Source: CAD feature listing. Evaluate the final solid. Frame: model axes, mm. A direction names the side the tool comes from. Give positions to 0.01 mm unless a question says otherwise; leave off trailing zeros. Write each loop counter-clockwise with the first axis right and the second up, starting at its lowest first coordinate (ties: lowest second). Pieces come first, ordered by that corner, then holes. Notation, with made-up numbers: (-19.75, 19.5) -> (27.25, 19.5) arc R19 cw to (27.25, 41.5) -> close; hole circle Ø2 at (16.25, 62). An arc over 180 degrees is marked (long way). Answer as a JSON object with one key per item and string values. Group by question number.
Item 1: First-contact query: pin 1 Ø4 at (x, z) = (10.26, -4.32) entering from +Y; pin 2 Ø17.5 at (x, z) = (-20, 9) entering from -Y; pin 3 Ø2 at (x, y) = (-0.5, 2.5) entering from +Z; pin 4 Ø6 at (y, z) = (-10, 9.5) entering from -X. Flat tips, straight axial feed; report the tip coordinate or a pass-through.
Item 2: Section query A-A on z = 0. Return the cut outline in (x, y).
Item 3: Access query for faces 5 (the face through (-16, 0, 12)), 6 (the face through (-11, 4, 18.368)), 7 (the face through (-15, 4, -9.832)), 8 (the face through (-16, 7.2, 12)). Directions: +Z, -Z, +X, -X, +Y, -Y. A direction counts if a zero-diameter tool reaches every point of the face in a straight line with its end or side. Return the directions, or none.
Item 4: Section query B-B on x = 2. Return the cut outline in (y, z), plus the area to 3 significant figures.
Item 5: Pull-direction query (X, two-part tool) for faces 1 (the face through (-35.136, 4, 1)), 2 (the face through (-15, 4, 11.168)), 3 (the face through (-11, 4, -16.632)), 4 (the face through (-45.2, 3.7, 15.7)); classes: pulls with the +X half, pulls with the -X half, needs draft (parallel to the pull), parting line crosses it, or undercut.
Item 6: Section query D-D on y = 5.5. Return the cut outline in (x, z).
Item 7: Section query C-C on y = -15. Return the cut outline in (x, z), plus the area to 3 significant figures.
Item 8: Ray query, probe 1 along Y at (x, z) = (19, 0); probe 2 along Z at (x, y) = (-5, 4.5); probe 3 along Z at (x, y) = (11.5, 5). Return the intervals inside material, ascending. Write a range as from..to.
from build123d import *

# Parameters (mm, degrees)
SKETCH1_W           = 65
SKETCH1_H           = 35
BOSS_EXTRUDE1_DEPTH = 7.2
FILLET1_R           = 9
SKETCH5_R           = 2.25
SKETCH5_R_2         = 0.8
CUT_EXTRUDE1_DEPTH  = 52.716073838
SKETCH7_R           = 35
BOSS_EXTRUDE2_DEPTH = 7
CUT_EXTRUDE3_REACH  = 89.651
SKETCH8_R           = 4.25
SKETCH8_R_2         = 1
CUT_EXTRUDE4_REACH  = 82.469
SKETCH9_R           = 2.192172412
SKETCH9_R_2         = 2.2
SKETCH9_W           = 41
SKETCH9_H           = 21


with BuildPart() as part:
    # Sketch1 → Boss-Extrude1 (new body)
    with BuildSketch(Plane(origin=(0, 0, 0), x_dir=(1, 0, 0), z_dir=(0, 1, 0))):
        with Locations((-15.305107108, -0.868016429)):
            Rectangle(SKETCH1_W, SKETCH1_H)
    extrude(amount=BOSS_EXTRUDE1_DEPTH)

    # Fillet1
    fillet1_edges = [part.edges().sort_by_distance(p)[0] for p in [
        (-47.805107108, 3.6, -16.631983571),
        (-47.805107108, 3.6, 18.368016429),
    ]]
    fillet(fillet1_edges, radius=FILLET1_R)

    # Sketch5 → Cut-Extrude1 (cut, through all)
    with BuildSketch(Plane(origin=(0, 7.2, 0), x_dir=(1, 0, 0), z_dir=(0, 1, 0))):
        with Locations(Location((-24.935816815, -0.668016429, 0), (0, 0, 270))):
            Circle(SKETCH5_R)
        with Locations(Location((-28.935816815, -0.669860131, 0), (0, 0, 270))):
            Circle(SKETCH5_R_2)
        with Locations(Location((-20.935816815, -0.669860131, 0), (0, 0, 270))):
            Circle(SKETCH5_R_2)
    extrude(amount=-CUT_EXTRUDE1_DEPTH, mode=Mode.SUBTRACT)

    # Sketch7 → Boss-Extrude2 (add)
    with BuildSketch(Plane(origin=(17.194892892, 0, 0), x_dir=(0, 0, -1), z_dir=(1, 0, 0))):
        with Locations((0, -12.251447975)):
            Circle(SKETCH7_R)
    extrude(amount=BOSS_EXTRUDE2_DEPTH)

    # Sketch8 → Cut-Extrude3 (cut, up to next)
    with BuildSketch(Plane.ZY.offset(-17.194892892), mode=Mode.PRIVATE) as cut_extrude3_sk1:
        with Locations((0, -12.251447975)):
            Circle(SKETCH8_R)
    cut_extrude3_tool1 = extrude(cut_extrude3_sk1.sketch, amount=-CUT_EXTRUDE3_REACH, mode=Mode.PRIVATE) & part.part
    # Sketch8 → Cut-Extrude3 (cut, up to next)
    with BuildSketch(Plane.ZY.offset(-17.194892892), mode=Mode.PRIVATE) as cut_extrude3_sk2:
        with Locations((-10.511534724, -12.874775935)):
            Circle(SKETCH8_R_2)
    cut_extrude3_tool2 = extrude(cut_extrude3_sk2.sketch, amount=-CUT_EXTRUDE3_REACH, mode=Mode.PRIVATE) & part.part
    # Sketch8 → Cut-Extrude3 (cut, up to next)
    with BuildSketch(Plane.ZY.offset(-17.194892892), mode=Mode.PRIVATE) as cut_extrude3_sk3:
        with Locations((10.511534724, -11.628120014)):
            Circle(SKETCH8_R_2)
    cut_extrude3_tool3 = extrude(cut_extrude3_sk3.sketch, amount=-CUT_EXTRUDE3_REACH, mode=Mode.PRIVATE) & part.part
    add(cut_extrude3_tool1.solids().sort_by_distance((17.194893, -12.251448, 0))[0], mode=Mode.SUBTRACT)
    add(cut_extrude3_tool2.solids().sort_by_distance((17.194893, -12.874776, -10.511535))[0], mode=Mode.SUBTRACT)
    add(cut_extrude3_tool3.solids().sort_by_distance((17.194893, -11.62812, 10.511535))[0], mode=Mode.SUBTRACT)

    # Sketch9 → Cut-Extrude4 (cut, up to next)
    with BuildSketch(Plane(origin=(0, 7.2, 0), x_dir=(1, 0, 0), z_dir=(0, 1, 0)), mode=Mode.PRIVATE) as cut_extrude4_sk1:
        with Locations(Location((10.257150233, 4.32491084, 0), (0, 0, 270))):
            Circle(SKETCH9_R)
    cut_extrude4_tool1 = extrude(cut_extrude4_sk1.sketch, amount=-CUT_EXTRUDE4_REACH, mode=Mode.PRIVATE) & part.part
    # Sketch9 → Cut-Extrude4 (cut, up to next)
    with BuildSketch(Plane(origin=(0, 7.2, 0), x_dir=(1, 0, 0), z_dir=(0, 1, 0)), mode=Mode.PRIVATE) as cut_extrude4_sk2:
        with Locations(Location((10.253796486, -5.668016429, 0), (0, 0, 270))):
            Circle(SKETCH9_R_2)
    cut_extrude4_tool2 = extrude(cut_extrude4_sk2.sketch, amount=-CUT_EXTRUDE4_REACH, mode=Mode.PRIVATE) & part.part
    # Sketch9 → Cut-Extrude4 (cut, up to next)
    with BuildSketch(Plane(origin=(0, 7.2, 0), x_dir=(1, 0, 0), z_dir=(0, 1, 0)), mode=Mode.PRIVATE) as cut_extrude4_sk3:
        with Locations(Location((-39.525430116, -5.668016429, 0), (0, 0, 270))):
            Circle(SKETCH9_R_2)
    cut_extrude4_tool3 = extrude(cut_extrude4_sk3.sketch, amount=-CUT_EXTRUDE4_REACH, mode=Mode.PRIVATE) & part.part
    # Sketch9 → Cut-Extrude4 (cut, up to next)
    with BuildSketch(Plane(origin=(0, 7.2, 0), x_dir=(1, 0, 0), z_dir=(0, 1, 0)), mode=Mode.PRIVATE) as cut_extrude4_sk4:
        with Locations(Location((-39.525430116, 4.331983571, 0), (0, 0, 270))):
            Circle(SKETCH9_R_2)
    cut_extrude4_tool4 = extrude(cut_extrude4_sk4.sketch, amount=-CUT_EXTRUDE4_REACH, mode=Mode.PRIVATE) & part.part
    # Sketch9 → Cut-Extrude4 (cut, up to next)
    with BuildSketch(Plane(origin=(0, 7.2, 0), x_dir=(1, 0, 0), z_dir=(0, 1, 0)), mode=Mode.PRIVATE) as cut_extrude4_sk5:
        with Locations((-14.635816815, -0.668016429)):
            Rectangle(SKETCH9_W, SKETCH9_H)
    cut_extrude4_tool5 = extrude(cut_extrude4_sk5.sketch, amount=-CUT_EXTRUDE4_REACH, mode=Mode.PRIVATE) & part.part
    add(cut_extrude4_tool1.solids().sort_by_distance((10.25715, 7.2, -4.324911))[0], mode=Mode.SUBTRACT)
    add(cut_extrude4_tool2.solids().sort_by_distance((10.253796, 7.2, 5.668016))[0], mode=Mode.SUBTRACT)
    add(cut_extrude4_tool3.solids().sort_by_distance((-39.52543, 7.2, 5.668016))[0], mode=Mode.SUBTRACT)
    add(cut_extrude4_tool4.solids().sort_by_distance((-39.52543, 7.2, -4.331984))[0], mode=Mode.SUBTRACT)
    add(cut_extrude4_tool5.solids().sort_by_distance((-14.635817, 7.2, 0.668016))[0], mode=Mode.SUBTRACT)


solid = part.part
Worked answers:
{
 "1": {"pin 1": "through", "pin 2": "y = 0", "pin 3": "z = 18.37", "pin 4": "x = 17.19"},
 "2": {"outline": "(-47.81, 0) -> (-35.14, 0) -> (-35.14, 7.2) -> (-47.81, 7.2) -> close; (5.86, 0) -> (17.19, 0) -> (17.19, -8) -> (24.19, -8) -> (24.19, 22.75) -> (17.19, 22.75) -> (17.19, 7.2) -> (5.86, 7.2) -> close; (17.19, -47.25) -> (24.19, -47.25) -> (24.19, -16.5) -> (17.19, -16.5) -> close"},
 "3": {"face 5": "+Z, -Z, -X, -Y", "face 6": "+Z, -X, +Y, -Y", "face 7": "+Y, -Y", "face 8": "+Z, -Z, -X, +Y"},
 "4": {"outline": "(0, -16.63) -> (7.2, -16.63) -> (7.2, -9.83) -> (0, -9.83) -> close; (0, 11.17) -> (7.2, 11.17) -> (7.2, 18.37) -> (0, 18.37) -> close", "area": "101 mm^2"},
 "5": {"face 1": "undercut", "face 2": "undercut", "face 3": "needs draft", "face 4": "pulls with the -X half"},
 "6": {"outline": "(-47.81, -7.63) arc R9 ccw to (-38.81, -16.63) -> (17.19, -16.63) -> (17.19, -30.16) -> (24.19, -30.16) -> (24.19, 30.16) -> (17.19, 30.16) -> (17.19, 18.37) -> (-38.81, 18.37) arc R9 ccw to (-47.81, 9.37) -> close; hole circle Ø4.4 at (-39.53, -4.33); hole circle Ø4.4 at (-39.53, 5.67); hole (-35.14, -9.83) -> (5.86, -9.83) -> (5.86, 11.17) -> (-35.14, 11.17) -> close; hole circle Ø4.4 at (10.25, 5.67); hole circle Ø4.38 at (10.26, -4.32)"},
 "7": {"outline": "(17.19, -34.89) -> (24.19, -34.89) -> (24.19, -3.24) -> (17.19, -3.24) -> close; (17.19, 3.24) -> (24.19, 3.24) -> (24.19, 34.89) -> (17.19, 34.89) -> close", "area": "443 mm^2"},
 "8": {"probe 1": "-47.25..-16.5, -8..22.75", "probe 2": "-16.63..-9.83, 11.17..18.37", "probe 3": "-16.63..-6.13, -2.52..3.86, 7.48..18.37"}
}
